from build123d import *

# Parameters (mm, degrees)
F1_DEPTH = 50.8


with BuildPart() as f1:
    # F0 (on Top) → F1 (new body)
    with BuildSketch(Plane.XY):
        Polygon((-101.6, 0), (0, 0), (0, 25.4), (0, 50.8), (0, 76.2), (-101.6, 76.2), align=None)
        Polygon((0, 50.8), (0, 25.4), (50.8, 0), (50.8, 75.968106), align=None)
    extrude(amount=-F1_DEPTH)


solid = f1.part
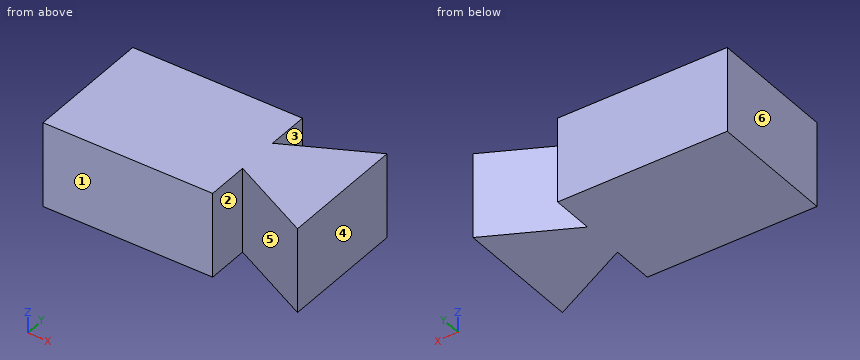
Geometry check sheet. Reference: the model listing, model coordinates, mm. Face numbers are marked on the shaded views. A direction names the side the tool comes from. Give positions to 0.01 mm unless a question says otherwise; leave off trailing zeros. Write each loop counter-clockwise with the first axis right and the second up, starting at its lowest first coordinate (ties: lowest second). Pieces come first, ordered by that corner, then holes.
1) Release check for a two-part mould opening along X. For the marked faces 4, 5 and 6 record: released by +X, released by -X, zero draft, split by the parting line, or undercut.
Values follow:
face 4: released by +X
face 5: undercut
face 6: released by -X
2) Cross-section at B-B (z = -33.5). Record the boundary of the cut face in (x, y), plus the area to 3 significant figures.
Values follow:
outline: (-101.6, 0) - (0, 0) - (0, 25.4) - (50.8, 0) - (50.8, 75.97) - (0, 50.8) - (0, 76.2) - (-101.6, 76.2) - close
area: 10,300 mm2
3) Cross-section at A-A (y = 65). Record the boundary of the cut face in (x, z).
Values follow:
outline: (-101.6, -50.8) - (0, -50.8) - (0, 0) - (-101.6, 0) - close; (28.66, -50.8) - (50.8, -50.8) - (50.8, 0) - (28.66, 0) - close
4) Set-up check for the marked faces 1, 2 and 3: record each of +Z, -Z, +X, -X, +Y, -Y from which the full face is reachable in a straight line by a thin tool's end or side.
Values follow:
face 1: +Z, -Z, +X, -X, -Y
face 2: +Z, -Z, -Y
face 3: +Z, -Z, +Y
5) Thickness scan on line 1 (X direction, y = 58, z = -8); line 2 (X direction, y = 7, z = -40); line 3 (Y direction, x = 12.5, z = -43). Record the ranges inside material, lowest first.
Values follow:
line 1: x = -101.6 to 0, 14.53 to 50.8
line 2: x = -101.6 to 0, 36.8 to 50.8
line 3: y = 19.15 to 56.99
6) Cross-section at C-C (x = 28). Record the boundary of the cut face in (y, z), plus the area to 3 significant figures.
Values follow:
outline: (11.4, -50.8) - (64.67, -50.8) - (64.67, 0) - (11.4, 0) - close
area: 2,710 mm2
7) Go/stop test with flat-tipped pins: pin 1 Ø1 at (x, z) = (6.5, -44.5) entering from -Y; pin 2 Ø3 at (x, y) = (26.5, 10) entering from -Z. Record where each tip stops, or that it passes through.
Values follow:
pin 1: stops at y = 21.9
pin 2: passes through
